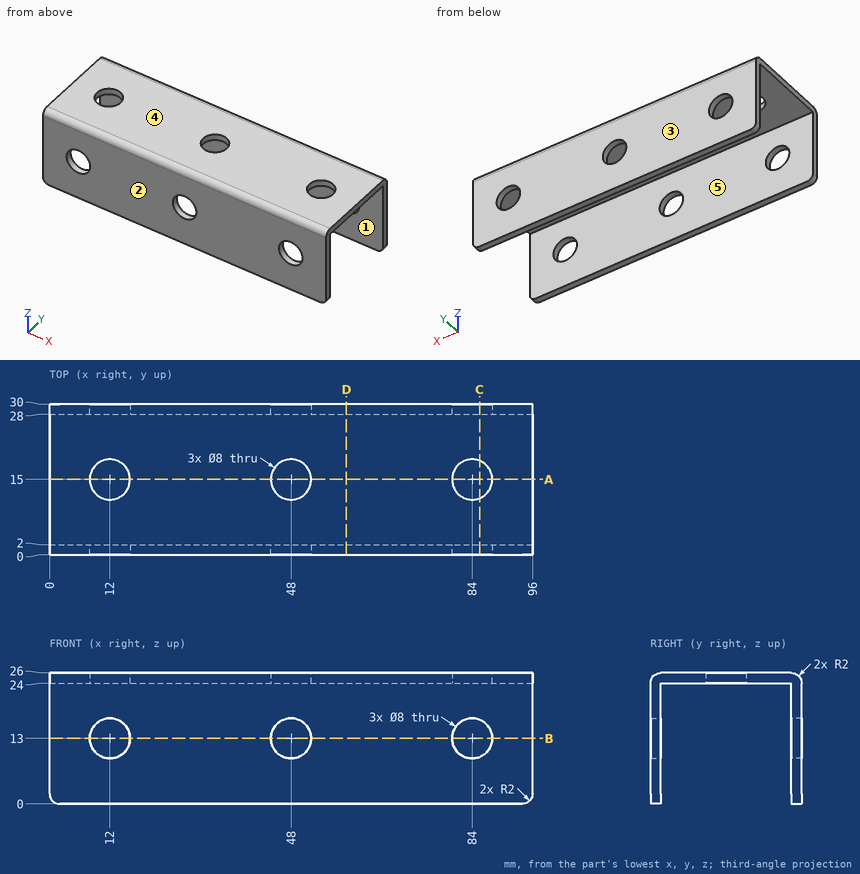
Verification items for this drawing (mm, ordinates from the low corner). A direction names the side the tool comes from. Round coordinates to 2 decimals unless told otherwise and drop trailing zeros. Loops run counter-clockwise (first coordinate to the right, second up) from the corner with the lowest first, then second, coordinate; pieces in that order, holes last. Notation, with made-up numbers: (72, 11) - (129, 11) arc R27 cw to (129, 31) - close; hole circle Ø1 at (37.5, -33.5). An arc over 180 degrees is marked (long way). Answer as CSV lines item,"result". Start each with the question number.
Item 1: Depth check by flat-ended pin: P1, Ø2, axis at x = 56.5, y = 5.5, coming from the -Z side; P2, Ø7, axis at x = 48, z = 13, coming from the +Y side. Enter the tip coordinate at first touch or a pass-through.
Item 2: Section check D-D (x = 59). Record the boundary of the cut face in (y, z).
Item 3: Section check C-C (x = 85.5). Record the boundary of the cut face in (y, z), and give its area (3 significant figures).
Item 4: Release check for a two-part mould opening along Y. For the marked faces 3, 4 and 5 record: +Y half, -Y half, draft (parallel to the pull), parting line (faces both ways), or undercut.
Item 5: Set-up check for the marked faces 1 and 2: record each of +Z, -Z, +X, -X, +Y, -Y from which the full face is reachable in a straight line by a thin tool's end or side.
Item 6: Section check B-B (z = 13). Count the separate pieces of the cut face and the enclosed holes in it, and give its area (3 significant figures).
Item 7: Section check A-A (y = 15). Record the boundary of the cut face in (x, z), and give its area (3 significant figures).
Item 8: Scan lines: line 1 (Y direction, x = 86, z = 7.5); line 2 (Z direction, x = 88.5, y = 3.5); line 3 (Y direction, x = 48, z = 24.75). Record each from-to range of solid material in increasing order. Write a range as [from, to].
Report:
1,P1,"stops at z = 24"
1,P2,"passes through"
2,outline,"(0, 0) - (2, 0) - (2, 24) - (28, 24) - (28, 0) - (30, 0) - (30, 24) arc R2 ccw to (28, 26) - (2, 26) arc R2 ccw to (0, 24) - close"
3,outline,"(0, 0) - (2, 0) - (2, 9.29) - (0, 9.29) - close; (0, 16.71) - (2, 16.71) - (2, 24) - (11.29, 24) - (11.29, 26) - (2, 26) arc R2 ccw to (0, 24) - close; (18.71, 24) - (28, 24) - (28, 16.71) - (30, 16.71) - (30, 24) arc R2 ccw to (28, 26) - (18.71, 26) - close; (28, 0) - (30, 0) - (30, 9.29) - (28, 9.29) - close"
3,area,"110 mm2"
4,face 3,"+Y half"
4,face 4,"draft"
4,face 5,"undercut"
5,face 1,"-Z, +X, -X"
5,face 2,"+Z, -Z, +X, -X, -Y"
6,separate pieces,"8"
6,enclosed holes,"0"
6,area,"288 mm2"
7,outline,"(0, 24) - (8, 24) - (8, 26) - (0, 26) - close; (16, 24) - (44, 24) - (44, 26) - (16, 26) - close; (52, 24) - (80, 24) - (80, 26) - (52, 26) - close; (88, 24) - (96, 24) - (96, 26) - (88, 26) - close"
7,area,"144 mm2"
8,line 1,"y = [0, 2], [28, 30]"
8,line 2,"z = [24, 26]"
8,line 3,"y = [0.15, 11], [19, 29.85]"
